For this review, take the finished solid that the model builds, in its own axes (mm). A direction names the side the tool comes from. Round coordinates to 2 decimals unless told otherwise and drop trailing zeros. Loops run counter-clockwise (first coordinate to the right, second up) from the corner with the lowest first, then second, coordinate; pieces in that order, holes last.
1) Take a section at A-A (y = 8.5). State the section outline as (x, z) points, then the cut area to 3 significant figures.
2) Take a section at B-B (x = -8). State the section outline as (y, z) points.
3) Insertion check: pin 1 (2.5 mm diameter, centred on y = 6.5, z = 7, fed in from -X); pin 2 (2.5 mm diameter, centred on y = 7, z = -5, fed in from -X); pin 3 (2 mm diameter, centred on x = 7.5, y = 1.5, fed in from +Z). Each pin has a flat end and moves straight along its axis. Give the tip position at first contact, or say it passes through.
4) Take a section at C-C (z = 0). State the section outline as (x, y) points, then the cut area to 3 significant figures.
5) Tool access review of faces 4 (the flat face through (0, -2, 0)), 5 (the flat face through (-4, 4, 0.85)), 6 (the flat face through (0.85, 4, 4)): name each direction out of +Z, -Z, +X, -X, +Y, -Y from which nothing blocks a thin tool from reaching the whole face with its end or side.
6) Mouldability with a two-part tool opening along X and no side actions: class faces 1 (the flat face through (-0.85, 4, 4)), 2 (the flat face through (-4, 4, -0.85)), 3 (the cylindrical face through (23.846, -0.986, -7.509)) as pulls with the +X half, pulls with the -X half, needs draft (parallel to the pull), parting line crosses it, or undercut.
7) Wall thickness on L1, parallel to Y at x = 15.5, z = -19.5; L2, parallel to Z at x = -5, y = 7.75; L3, parallel to X at y = 1.25, z = 5: over which ranges is each line inside the solid? List them lowest first.
8) Take a section at D-D (y = 2.5). State the section outline as (x, z) points.
```python
from build123d import *

# Parameters (mm, degrees)
SKETCH1_R           = 25
BOSS_EXTRUDE1_DEPTH = 2
REVOLVE3_ANGLE      = 180
SKETCH7_W           = 1.7
SKETCH7_H           = 1.7
SKETCH7_W_2         = 9.15
SKETCH7_H_2         = 9.15
CUT_EXTRUDE1_DEPTH  = 10


with BuildPart() as part:
    # Sketch1 → Boss-Extrude1 (new body)
    with BuildSketch(Plane(origin=(0, 0, 0), x_dir=(1, 0, 0), z_dir=(0, 1, 0))):
        Circle(SKETCH1_R)
    extrude(amount=-BOSS_EXTRUDE1_DEPTH)

    # Sketch6 → Revolve3 (revolve)
    with BuildSketch(Plane(origin=(0, 0, 0), x_dir=(1, 0, 0), z_dir=(0, 1, 0))):
        with BuildLine():
            Line((-10, 0), (10, 0))
            ThreePointArc((10, 0), (0, 10), (-10, 0))
        make_face()
    revolve(axis=Axis((-10, 0, 0), (1, 0, 0)), revolution_arc=REVOLVE3_ANGLE)

    # Sketch7 → Cut-Extrude1 (cut)
    with BuildSketch(Plane(origin=(0, 0, 0), x_dir=(1, 0, 0), z_dir=(0, 1, 0))):
        Rectangle(SKETCH7_W, SKETCH7_H)
        with Locations((-5.425, 0)):
            Rectangle(SKETCH7_W_2, SKETCH7_H)
        with Locations((0, 5.425)):
            Rectangle(SKETCH7_W, SKETCH7_H_2)
        with Locations((5.425, 0)):
            Rectangle(SKETCH7_W_2, SKETCH7_H)
        with Locations((0, -5.425)):
            Rectangle(SKETCH7_W, SKETCH7_H_2)
    extrude(amount=CUT_EXTRUDE1_DEPTH, mode=Mode.SUBTRACT)


solid = part.part
```
Response:
1. outline: (-5.2, -0.85) arc R5.27 ccw to (-0.85, -5.2) - (-0.85, -0.85) - close; (-5.2, 0.85) - (-0.85, 0.85) - (-0.85, 5.2) arc R5.27 ccw to start; (0.85, -5.2) arc R5.27 ccw to (5.2, -0.85) - (0.85, -0.85) - close; (0.85, 0.85) - (5.2, 0.85) arc R5.27 ccw to (0.85, 5.2) - close
1. area: 54.4 mm2
2. outline: (-2, -23.69) - (0, -23.69) - (0, -6) arc R6 ccw to (5.94, -0.85) - (0, -0.85) - (0, 0.85) - (5.94, 0.85) arc R6 ccw to (0, 6) - (0, 23.69) - (-2, 23.69) - close
3. pin 1: stops at x = -5.57
3. pin 2: stops at x = -6.78
3. pin 3: stops at z = 7.47
4. outline: (-25, -2) - (25, -2) - (25, 0) - (-25, 0) - close
4. area: 100 mm2
5. face 4: +Z, -Z, +X, -X, -Y
5. face 5: +X, -X, +Y
5. face 6: +Z, -Z, +Y
6. face 1: undercut
6. face 2: needs draft
6. face 3: parting line crosses it
7. L1: y = -2 to 0
7. L2: z = -3.86 to -0.85, 0.85 to 3.86
7. L3: x = -8.57 to -0.85, 0.85 to 8.57
8. outline: (-9.65, -0.85) arc R9.68 ccw to (-0.85, -9.65) - (-0.85, -0.85) - close; (-9.65, 0.85) - (-0.85, 0.85) - (-0.85, 9.65) arc R9.68 ccw to start; (0.85, -9.65) arc R9.68 ccw to (9.65, -0.85) - (0.85, -0.85) - close; (0.85, 0.85) - (9.65, 0.85) arc R9.68 ccw to (0.85, 9.65) - close
